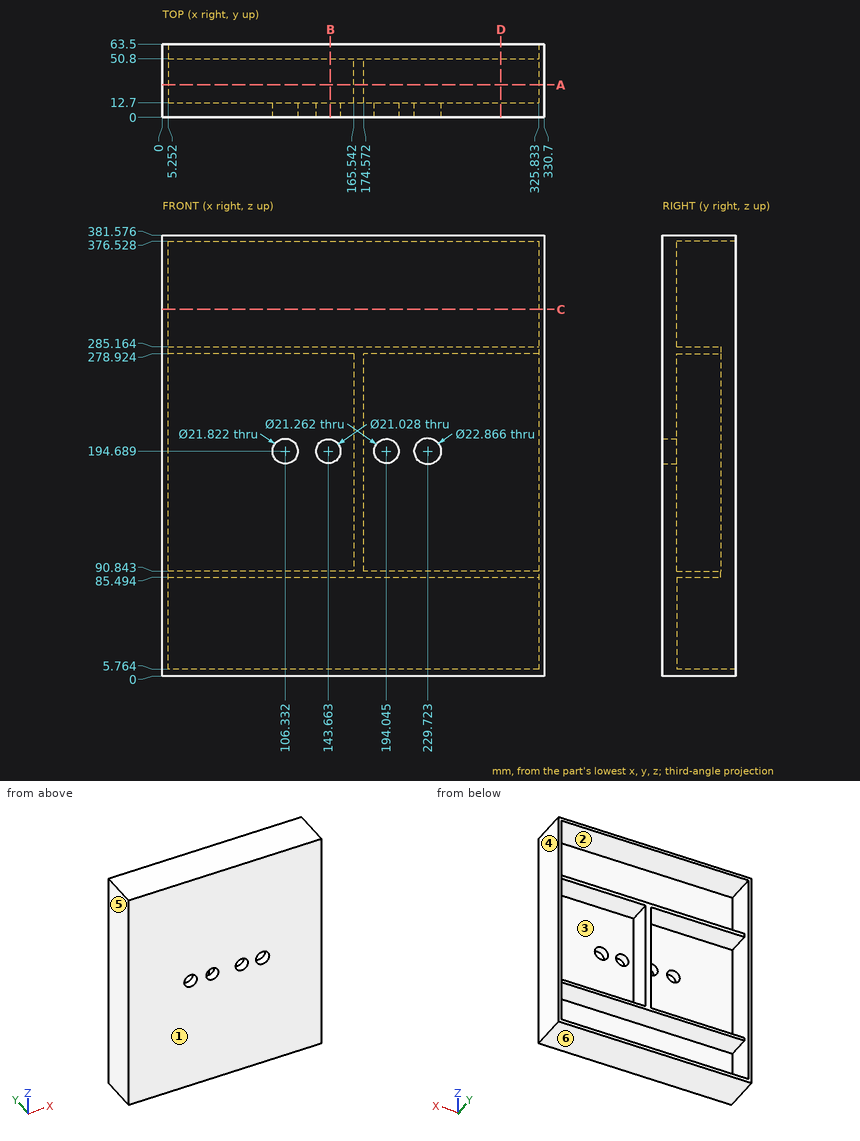
Part print with two shaded views. Sizes in mm from the minimum x, y, z corner. A direction names the side the tool comes from. Round coordinates to 2 decimals unless told otherwise and drop trailing zeros. Loops run counter-clockwise (first coordinate to the right, second up) from the corner with the lowest first, then second, coordinate; pieces in that order, holes last.
Item 1: Saw through at A-A (y = 28). List the corners of the cut face in (x, z) (1 decimal), then the cut area to 3 significant figures.
Item 2: Pin check, flat tips, straight feed: P1, Ø1, axis at x = 40.5, z = 275.5, coming from the +Y side; P2, Ø20.5, axis at x = 229.72, z = 194.69, coming from the -Y side. Stop position of each tip, or through.
Item 3: Two-plate mould, pull along X, no slides. Class the marked faces 3, 4, 5 and 6: released by +X, released by -X, zero draft, split by the parting line, or undercut.
Item 4: Saw through at D-D (x = 293). List the corners of the cut face in (y, z) (1 decimal).
Item 5: Saw through at C-C (z = 317.5). List the corners of the cut face in (x, y).
Item 6: Which spindle directions (+Z, -Z, +X, -X, +Y, -Y) get a long thin tool onto all of the face, cutting with end or side? Do the marked faces 1 and 2. Say none if no direction does.
Item 7: Saw through at B-B (x = 145.5). List the corners of the cut face in (y, z) (1 decimal).
Item 8: Drill centre lines: line 1 along X through (y, z) = (24, 214); line 2 along Z through (x, y) = (100, 49) (1 decimal); line 3 along Z through (x, y) = (279, 58.5) (1 decimal). Where is each one in solid material? Low to high.
Worked answers:
1. outline: (0, 0) - (330.7, 0) - (330.7, 381.6) - (0, 381.6) - close; hole (5.3, 5.8) - (325.8, 5.8) - (325.8, 85.5) - (5.3, 85.5) - close; hole (5.3, 90.8) - (165.5, 90.8) - (165.5, 278.9) - (5.3, 278.9) - close; hole (5.3, 285.2) - (325.8, 285.2) - (325.8, 376.5) - (5.3, 376.5) - close; hole (174.6, 90.8) - (325.8, 90.8) - (325.8, 278.9) - (174.6, 278.9) - close
1. area: 12,700 mm2
2. P1: stops at y = 12.7
2. P2: passes through
3. face 3: undercut
3. face 4: released by +X
3. face 5: released by -X
3. face 6: zero draft
4. outline: (0, 0) - (63.5, 0) - (63.5, 5.8) - (12.7, 5.8) - (12.7, 85.5) - (50.8, 85.5) - (50.8, 90.8) - (12.7, 90.8) - (12.7, 278.9) - (50.8, 278.9) - (50.8, 285.2) - (12.7, 285.2) - (12.7, 376.5) - (63.5, 376.5) - (63.5, 381.6) - (0, 381.6) - close
5. outline: (0, 0) - (330.7, 0) - (330.7, 63.5) - (325.83, 63.5) - (325.83, 12.7) - (5.25, 12.7) - (5.25, 63.5) - (0, 63.5) - close
6. face 1: +Z, -Z, +X, -X, -Y
6. face 2: +Y
7. outline: (0, 0) - (63.5, 0) - (63.5, 5.8) - (12.7, 5.8) - (12.7, 85.5) - (50.8, 85.5) - (50.8, 90.8) - (12.7, 90.8) - (12.7, 184.3) - (0, 184.3) - close; (0, 205) - (12.7, 205) - (12.7, 278.9) - (50.8, 278.9) - (50.8, 285.2) - (12.7, 285.2) - (12.7, 376.5) - (63.5, 376.5) - (63.5, 381.6) - (0, 381.6) - close
8. line 1: x = 0 to 5.25, 165.54 to 174.57, 325.83 to 330.7
8. line 2: z = 0 to 5.8, 85.5 to 90.8, 278.9 to 285.2, 376.5 to 381.6
8. line 3: z = 0 to 5.8, 376.5 to 381.6
